The listing builds one solid part. Answer for the finished solid, in the listing's coordinates (mm). A direction names the side the tool comes from. Coordinates: 2 decimals unless noted, no trailing zeros. Loops run counter-clockwise (first coordinate to the right, second up) from the corner with the lowest first, then second, coordinate; pieces in that order, holes last. Notation, with made-up numbers: (5, 51.5) - (36, 51.5) arc R33 ccw to (36, 88.5) - close; hole circle Ø2 at (-15, -17). An arc over 180 degrees is marked (long way). Put each result on its own line as item: value.
```python
from build123d import *

# Parameters (mm, degrees)
SKETCH1_W            = 34.5
SKETCH1_H            = 40
BOSS_EXTRUDE1_DEPTH  = 26.3
FILLET1_R            = 1.5
SKETCH2_R            = 4.15
SKETCH2_R_2          = 3
BOSS_EXTRUDE2_DEPTH  = 14.2
SKETCH3_R            = 4.15
SKETCH3_R_2          = 3
BOSS_EXTRUDE3_DEPTH  = 3
BOSS_EXTRUDE3_DRAFT  = 14
SKETCH4_R            = 4.15
BOSS_EXTRUDE4_DEPTH  = 3
BOSS_EXTRUDE4_DRAFT  = -14
SKETCH5_R            = 4.15
SKETCH5_R_2          = 3
BOSS_EXTRUDE5_DEPTH  = 15.6
SKETCH6_R            = 6.15
BOSS_EXTRUDE6_DEPTH  = 1.7
FILLET2_R            = 2
SKETCH7_R            = 4.15
SKETCH7_R_2          = 3
BOSS_EXTRUDE7_DEPTH  = 3
BOSS_EXTRUDE7_DRAFT  = 14
SKETCH8_R            = 4.15
BOSS_EXTRUDE8_DEPTH  = 3
BOSS_EXTRUDE8_DRAFT  = -14
BOSS_EXTRUDE9_DEPTH  = 3
SKETCH10_W           = 10.5
SKETCH10_H           = 15.2
SKETCH10_R           = 1.5
BOSS_EXTRUDE10_DEPTH = 2
SKETCH11_W           = 1.5
SKETCH11_H           = 15.2
BOSS_EXTRUDE11_DEPTH = 36
BOSS_EXTRUDE12_DEPTH = 1.5
BOSS_EXTRUDE14_START = -1.5
BOSS_EXTRUDE14_DEPTH = 1.5


with BuildPart() as part:
    # Sketch1 → Boss-Extrude1 (new body)
    with BuildSketch(Plane.XY):
        Rectangle(SKETCH1_W, SKETCH1_H)
    extrude(amount=BOSS_EXTRUDE1_DEPTH)

    # Fillet1
    fillet1_edges = [part.edges().sort_by_distance(p)[0] for p in [
        (17.25, 0, 26.3),
        (-17.25, 0, 26.3),
        (17.25, 0, 0),
        (-17.25, 0, 0),
    ]]
    fillet(fillet1_edges, radius=FILLET1_R)

    # Sketch2 → Boss-Extrude2 (add)
    with BuildSketch(Plane(origin=(0, 20, 0), x_dir=(1, 0, 0), z_dir=(0, 1, 0))):
        with Locations(Location((-5.712581949, -13.35, 0), (0, 0, 270))):
            Circle(SKETCH2_R)
        with Locations(Location((-5.712581949, -13.35, 0), (0, 0, 270))):
            Circle(SKETCH2_R_2, mode=Mode.SUBTRACT)
    extrude(amount=BOSS_EXTRUDE2_DEPTH)


with BuildPart() as boss_extrude3_tool:
    # Sketch3 → Boss-Extrude3 (with draft: the straight prism first)
    with BuildSketch(Plane(origin=(0, 34.2, 0), x_dir=(1, 0, 0), z_dir=(0, 1, 0))):
        with Locations(Location((-5.712581949, -13.35, 0), (0, 0, 270))):
            Circle(SKETCH3_R)
        with Locations(Location((-5.712581949, -13.35, 0), (0, 0, 270))):
            Circle(SKETCH3_R_2, mode=Mode.SUBTRACT)
    extrude(amount=-BOSS_EXTRUDE3_DEPTH)
    # Boss-Extrude3: the draft: its side faces are tilted about the plane it starts from
    boss_extrude3_sides = [boss_extrude3_tool.faces().sort_by_distance(p)[0] for p in [
        (-5.712581949, 32.7, 9.2),
        (-5.712581949, 32.7, 10.35),
    ]]
    draft(boss_extrude3_sides, Plane(origin=(0, 34.2, 0), x_dir=(1, 0, 0), z_dir=(0, 1, 0)), BOSS_EXTRUDE3_DRAFT)


with BuildPart() as part_1:
    add(part.part)

    # Boss-Extrude3: add boss_extrude3_tool
    add(boss_extrude3_tool.part)


with BuildPart() as boss_extrude4_tool:
    # Sketch4 → Boss-Extrude4 (with draft: the straight prism first)
    with BuildSketch(Plane.XZ.offset(-31.2)):
        with Locations(Location((-5.712581949, 13.35, 0), (0, 0, 270))):
            Circle(SKETCH4_R)
    extrude(amount=BOSS_EXTRUDE4_DEPTH)
    # Boss-Extrude4: the draft: its side faces are tilted about the plane it starts from
    boss_extrude4_sides = [boss_extrude4_tool.faces().sort_by_distance(p)[0] for p in [
        (-5.712581949, 29.7, 17.5),
    ]]
    draft(boss_extrude4_sides, Plane.XZ.offset(-31.2), BOSS_EXTRUDE4_DRAFT)


with BuildPart() as part_2:
    add(part_1.part)

    # Boss-Extrude4: add boss_extrude4_tool
    add(boss_extrude4_tool.part)

    # Sketch5 → Boss-Extrude5 (add)
    with BuildSketch(Plane.XY.offset(26.3)):
        with Locations(Location((5.1, 11.85, 0), (0, 0, 180))):
            Circle(SKETCH5_R)
        with Locations((5.1, 11.85)):
            Circle(SKETCH5_R_2, mode=Mode.SUBTRACT)
    extrude(amount=BOSS_EXTRUDE5_DEPTH)

    # Sketch6 → Boss-Extrude6 (add)
    with BuildSketch(Plane.XY.offset(26.3)):
        with Locations(Location((5.1, 11.85, 0), (0, 0, 180))):
            Circle(SKETCH6_R)
    extrude(amount=BOSS_EXTRUDE6_DEPTH)

    # Fillet2
    fillet2_edges = [part_2.edges().sort_by_distance(p)[0] for p in [
        (-5.712581949, 20, 9.2),
        (9.25, 11.85, 28),
    ]]
    fillet(fillet2_edges, radius=FILLET2_R - 0.0001)  # a hair under: the kernel refuses the full size


with BuildPart() as boss_extrude7_tool:
    # Sketch7 → Boss-Extrude7 (with draft: the straight prism first)
    with BuildSketch(Plane.XY.offset(41.9)):
        with Locations((5.1, 11.85)):
            Circle(SKETCH7_R)
        with Locations((5.1, 11.85)):
            Circle(SKETCH7_R_2, mode=Mode.SUBTRACT)
    extrude(amount=-BOSS_EXTRUDE7_DEPTH)
    # Boss-Extrude7: the draft: its side faces are tilted about the plane it starts from
    boss_extrude7_sides = [boss_extrude7_tool.faces().sort_by_distance(p)[0] for p in [
        (0.95, 11.85, 40.4),
        (2.1, 11.85, 40.4),
    ]]
    draft(boss_extrude7_sides, Plane.XY.offset(41.9), BOSS_EXTRUDE7_DRAFT)


with BuildPart() as part_3:
    add(part_2.part)

    # Boss-Extrude7: add boss_extrude7_tool
    add(boss_extrude7_tool.part)


with BuildPart() as boss_extrude8_tool:
    # Sketch8 → Boss-Extrude8 (with draft: the straight prism first)
    with BuildSketch(Plane(origin=(0, 0, 38.9), x_dir=(-1, 0, 0), z_dir=(0, 0, -1))):
        with Locations((-5.1, 11.85)):
            Circle(SKETCH8_R)
    extrude(amount=BOSS_EXTRUDE8_DEPTH)
    # Boss-Extrude8: the draft: its side faces are tilted about the plane it starts from
    boss_extrude8_sides = [boss_extrude8_tool.faces().sort_by_distance(p)[0] for p in [
        (9.25, 11.85, 37.4),
    ]]
    draft(boss_extrude8_sides, Plane(origin=(0, 0, 38.9), x_dir=(-1, 0, 0), z_dir=(0, 0, -1)), BOSS_EXTRUDE8_DRAFT)


with BuildPart() as part_4:
    add(part_3.part)

    # Boss-Extrude8: add boss_extrude8_tool
    add(boss_extrude8_tool.part)

    # Sketch9 → Boss-Extrude9 (add)
    with BuildSketch(Plane.XZ.offset(20)):
        with BuildLine():
            Line((-13.4, 4.074600211), (-17.25, 4.074600211))
            Line((-17.25, 4.074600211), (-17.25, 8.374600211))
            Line((-17.25, 8.374600211), (-13.4, 8.374600211))
            ThreePointArc((-13.4, 8.374600211), (-11.25, 6.224600211), (-13.4, 4.074600211))
        make_face()
    extrude(amount=BOSS_EXTRUDE9_DEPTH)

    # Sketch10 → Boss-Extrude10 (add)
    # profile 1 of 2: a face of its own
    with BuildSketch(Plane(origin=(0, 0, 0), x_dir=(-1, 0, 0), z_dir=(0, 0, -1))):
        with Locations((22.5, 2.4)):
            Rectangle(SKETCH10_W, SKETCH10_H)
        with Locations((24.666201251, 2.4)):
            Circle(SKETCH10_R, mode=Mode.SUBTRACT)
    # profile 2 of 2: a face of its own
    with BuildSketch(Plane(origin=(0, 0, 0), x_dir=(-1, 0, 0), z_dir=(0, 0, -1))):
        with Locations((-22.5, 2.4)):
            Rectangle(SKETCH10_W, SKETCH10_H)
        with Locations((-24.285549997, 2.4)):
            Circle(SKETCH10_R, mode=Mode.SUBTRACT)
    extrude(amount=-BOSS_EXTRUDE10_DEPTH)

    # Sketch11 → Boss-Extrude11 (add)
    with BuildSketch(Plane(origin=(-17.25, 0, 0), x_dir=(0, 0, -1), z_dir=(1, 0, 0))):
        with Locations((-0.75, 2.4)):
            Rectangle(SKETCH11_W, SKETCH11_H)
    extrude(amount=BOSS_EXTRUDE11_DEPTH)

    # Sketch12 → Boss-Extrude12 (add)
    with BuildSketch(Plane.XZ.offset(5.2)):
        with BuildLine():
            Line((-17.25, 13.15), (-17.25, 2))
            Line((-17.25, 2), (-27.75, 2))
            ThreePointArc((-27.75, 2), (-21.157033541, 6.310323065), (-17.25, 13.15))
        make_face()
        with BuildLine():
            Line((17.25, 2), (27.75, 2))
            ThreePointArc((27.75, 2), (21.157033541, 6.310323065), (17.25, 13.15))
            Line((17.25, 13.15), (17.25, 2))
        make_face()
    extrude(amount=-BOSS_EXTRUDE12_DEPTH)

    # Sketch13 → Boss-Extrude14 (add)
    with BuildSketch(Plane(origin=(0, 10, 0), x_dir=(1, 0, 0), z_dir=(0, 1, 0)).offset(BOSS_EXTRUDE14_START)):
        with BuildLine():
            Line((-17.25, -13.15), (-17.25, -2))
            Line((-17.25, -2), (-27.75, -2))
            ThreePointArc((-27.75, -2), (-21.157033541, -6.310323065), (-17.25, -13.15))
        make_face()
        with BuildLine():
            Line((27.75, -2), (17.25, -2))
            Line((17.25, -2), (17.25, -13.15))
            ThreePointArc((17.25, -13.15), (21.157033541, -6.310323065), (27.75, -2))
        make_face()
    extrude(amount=BOSS_EXTRUDE14_DEPTH)


solid = part_4.part
```
1) The part is cut by section D-D (x = 21.5). Give the vertices of the cut face in (y, z), and give its area (3 significant figures).
Found:
outline: (-5.2, 0) - (10, 0) - (10, 5.96) - (8.5, 5.96) - (8.5, 2) - (-3.7, 2) - (-3.7, 5.96) - (-5.2, 5.96) - close
area: 42.3 mm^2
2) Each of these flat-tipped pins is pushed along its axis until it touches: pin 1 (2 mm diameter, centred on y = 11, z = 32, fed in from +X); pin 2 (2 mm diameter, centred on y = 9, z = 8, fed in from -X); pin 3 (5 mm diameter, centred on x = 24.29, y = 2.4, fed in from +Z). Where does it stop, or does it pass through?
Found:
pin 1: stops at x = 9.25
pin 2: stops at x = -20.54
pin 3: stops at z = 2
3) For a pull along Z with two mould halves and no side action, classify faces 5 (the face through (5, 12, 38.9)), 6 (the face through (0, -20, 13)), 7 (the face through (-6, 31.2, 13)), 8 (the face through (4.709, 14.824, 31.895)) as pulls with the +Z half, pulls with the -Z half, needs draft (parallel to the pull), parting line crosses it, or undercut.
Found:
face 5: pulls with the +Z half
face 6: needs draft
face 7: undercut
face 8: undercut
4) Straight lines are drawn through the part: L1, parallel to X at y = 23.5, z = 13.35; L2, parallel to Y at x = 5.1, z = 31.5; L3, parallel to X at y = -15, z = 22.5. For each, find the intervals that lie inside material, in ascending order. Write a range as [from, to].
Found:
L1: x = [-9.86, -8.71], [-2.71, -1.56]
L2: y = [7.7, 8.85], [14.85, 16]
L3: x = [-17.25, 17.25]
5) For faces 1 (the face through (-17.25, -2, 13)), 2 (the face through (-15, -21, 4.075)), 3 (the face through (17.25, 0, 13)), 4 (the face through (-2, 28.2, 16)), determine the directions among +Z, -Z, +X, -X, +Y, -Y from which every point of the face is accessible in a straight line to the end or side of a thin tool.
Found:
face 1: +Z, -X
face 2: -Z, +X, -X, -Y
face 3: +Z, +X
face 4: none
6) The part is cut by section C-C (z = 20.5). Give the vertices of the cut face in (x, y).
Found:
outline: (-17.25, -20) - (17.25, -20) - (17.25, 20) - (-17.25, 20) - close
